Part model, mm, in its own coordinate system. A direction names the side the tool comes from. Give positions to 0.01 mm unless a question says otherwise; leave off trailing zeros. Order: outer loops, then holes, each group sorted by start corner. A loop starts at its lowest first (then second) coordinate and runs counter-clockwise, first axis right, second up. Notation, with made-up numbers: (-36, -9.5) - (-17, -9.5) arc R31 cw to (-17, 29.5) - close; hole circle Ø8 at (81, 28). An arc over 180 degrees is marked (long way). One line per item, written item: value.
```python
from build123d import *

# Parameters (mm, degrees)
BOSS_EXTRUDE1_DEPTH = 12
SKETCH2_R           = 7.5
CUT_EXTRUDE1_DEPTH  = 120.620232402


with BuildPart() as part:
    # Sketch1 → Boss-Extrude1 (new body)
    with BuildSketch(Plane(origin=(0, 0, 0), x_dir=(0, 0, -1), z_dir=(1, 0, 0))):
        with BuildLine():
            Line((73, 94), (25, 94))
            Line((25, 94), (25, 65.097722286))
            ThreePointArc((25, 65.097722286), (25.604754635, 62.714065813), (27.272727273, 60.90702026))
            ThreePointArc((27.272727273, 60.90702026), (0, -31), (-27.272727273, 60.90702026))
            ThreePointArc((-27.272727273, 60.90702026), (-25.604754635, 62.714065813), (-25, 65.097722286))
            Line((-25, 65.097722286), (-25, 94))
            Line((-25, 94), (-73, 94))
            Line((-73, 94), (-73, -94))
            Line((-73, -94), (73, -94))
            Line((73, -94), (73, 94))
        make_face()
    extrude(amount=BOSS_EXTRUDE1_DEPTH)

    # Sketch2 → Cut-Extrude1 (cut, through all)
    with BuildSketch(Plane(origin=(12, 0, 0), x_dir=(0, 0, -1), z_dir=(1, 0, 0))):
        with Locations((43, -32)):
            Circle(SKETCH2_R)
    extrude(amount=-CUT_EXTRUDE1_DEPTH, mode=Mode.SUBTRACT)


solid = part.part
```
1) Which spindle directions (+Z, -Z, +X, -X, +Y, -Y) get a long thin tool onto all of the face, cutting with end or side? Do faces 5 (the flat face through (6, 94, 49)), 6 (the flat face through (6, 79, 25)), 7 (the cylindrical face through (5.92, 62.74, -25.59)). Say none if no direction does.
Outcome:
face 5: +Z, -Z, +X, -X, +Y
face 6: +X, -X, +Y
face 7: +X, -X
2) Mould opens along Z. For faces 1 (the flat face through (6, 94, -49)), 2 (the cylindrical face through (5.916, -30.968, -1.795)), 3 (the flat face through (6, -1, -73)), 4 (the flat face through (6, 1, 73)) say: released by +Z, released by -Z, zero draft, split by the parting line, or undercut.
Outcome:
face 1: zero draft
face 2: undercut
face 3: released by -Z
face 4: released by +Z
3) Cut at A-A, the plane y = 78.5. Give the cut face in (x, z), then the cut area to 3 significant figures.
Outcome:
outline: (0, -73) - (12, -73) - (12, -25) - (0, -25) - close; (0, 25) - (12, 25) - (12, 73) - (0, 73) - close
area: 1,150 mm^2
4) Drill centre lines: line 1 along Z through (x, y) = (3.25, 19); line 2 along Y through (x, z) = (7, -43); line 3 along Z through (x, y) = (3.75, 74). Where is each one in solid material? Low to high. Write a range as from..to.
Outcome:
line 1: z = -73..-50, 50..73
line 2: y = -94..-39.5, -24.5..-6.51, 44.51..94
line 3: z = -73..-25, 25..73
5) Cut at B-B, the plane x = 2. Give the cut face in (y, z), then the cut area to 3 significant figures.
Outcome:
outline: (-94, -73) - (94, -73) - (94, -25) - (65.1, -25) arc R5 ccw to (60.91, -27.27) arc R50 cw (long way) to (60.91, 27.27) arc R5 ccw to (65.1, 25) - (94, 25) - (94, 73) - (-94, 73) - close; hole circle Ø15 at (-32, -43)
area: 18,100 mm^2
6) Cut at C-C, the plane z = -43. Give the cut face in (x, y), then the cut area to 3 significant figures.
Outcome:
outline: (0, -94) - (12, -94) - (12, -39.5) - (0, -39.5) - close; (0, -24.5) - (12, -24.5) - (12, -6.51) - (0, -6.51) - close; (0, 44.51) - (12, 44.51) - (12, 94) - (0, 94) - close
area: 1,460 mm^2
7) Pin check, flat tip, straight feed: pin 1 (8 mm diameter, centred on y = 53, z = -29.5, fed in from -X). Stop position of the tip, or through.
Outcome:
pin 1: passes through
8) Cut at D-D, the plane y = 19. Give the cut face in (x, z), then the cut area to 3 significant figures.
Outcome:
outline: (0, -73) - (12, -73) - (12, -50) - (0, -50) - close; (0, 50) - (12, 50) - (12, 73) - (0, 73) - close
area: 552 mm^2
